```python
from build123d import *

# Parameters (mm, degrees)
SKETCH1_R           = 50
BOSS_EXTRUDE2_DEPTH = 10
SKETCH7_R           = 10.430903113
CUT_EXTRUDE5_DEPTH  = 10
CUT_EXTRUDE8_DEPTH  = 72.414284285
CUT_EXTRUDE9_DEPTH  = 72.414284285
CIRPATTERN3_COUNT   = 9
CIRPATTERN3_ANGLE   = 88
CIRPATTERN4_COUNT   = 17
CIRPATTERN4_ANGLE   = 176
SCALE3_SCALE        = 0.75
BOSS_EXTRUDE3_DEPTH = 15
BOSS_EXTRUDE6_DEPTH = 25
SKETCH19_R          = 1.5
CUT_EXTRUDE10_DEPTH = 2.5


with BuildPart() as part:
    # Sketch1 → Boss-Extrude2 (new body)
    with BuildSketch(Plane.YZ):
        with Locations(Location((0, 0, 0), (0, 0, 270))):
            Circle(SKETCH1_R)
    extrude(amount=BOSS_EXTRUDE2_DEPTH)

    # Sketch7 → Cut-Extrude5 (cut)
    with BuildSketch(Plane.YZ.offset(10)):
        with Locations(Location((0, 0, 0), (0, 0, 270))):
            Circle(SKETCH7_R)
    extrude(amount=-CUT_EXTRUDE5_DEPTH, mode=Mode.SUBTRACT)

    # Sketch10 → Cut-Extrude8 (cut, through all)
    with BuildSketch(Plane.YZ.offset(10)):
        with BuildLine():
            Line((-43.954399928, 0), (-14.132830655, 0))
            ThreePointArc((-14.132830655, 0), (10.058249892, -10.149932648), (0.129658997, 14.132830655))
            Line((0.129658997, 14.132830655), (0, 44.213717922))
            ThreePointArc((0, 44.213717922), (31.393478761, -30.950795255), (-43.954399928, 0))
        make_face()
    extrude(amount=-CUT_EXTRUDE8_DEPTH, mode=Mode.SUBTRACT)

    # Sketch12 → Cut-Extrude9 (cut, through all)
    with BuildSketch(Plane.YZ.offset(10)):
        Polygon((47.400317311, 0), (47.400317311, 0.608013975), (44.136400392, 2.742660057), (44.128376975, -2.615132262), (47.400317311, -0.500577082), align=None)
    cut_extrude9 = extrude(amount=-CUT_EXTRUDE9_DEPTH, mode=Mode.SUBTRACT)

    # CirPattern3: Cut-Extrude9 ×9 about axis
    cirpattern3_axis = Axis((0, 0.129658997, 0.129658997), (1, 0, 0))
    for i in range(1, CIRPATTERN3_COUNT):
        add(cut_extrude9.rotate(cirpattern3_axis, i * CIRPATTERN3_ANGLE / (CIRPATTERN3_COUNT - 1)), mode=Mode.SUBTRACT)

    # CirPattern4: Cut-Extrude9 ×17 about axis
    cirpattern4_axis = Axis((0, 0.129658997, 0.129658997), (-1, 0, 0))
    for i in range(1, CIRPATTERN4_COUNT):
        add(cut_extrude9.rotate(cirpattern4_axis, i * CIRPATTERN4_ANGLE / (CIRPATTERN4_COUNT - 1)), mode=Mode.SUBTRACT)


with BuildPart() as part_1:
    # Scale3: scaled about (0, 0, 0)
    add(part.part.scale(SCALE3_SCALE))

    # Sketch15 → Boss-Extrude3 (add)
    with BuildSketch(Plane.YZ.offset(7.5)):
        Polygon((-12.172757091, 41.059305133), (-7.956454872, 36.843002914), (-36.24072612, 8.558731667), (-40.457028339, 12.775033886), align=None)
    extrude(amount=BOSS_EXTRUDE3_DEPTH)

    # Sketch20 → Boss-Extrude6 (add)
    with BuildSketch(Plane(origin=(7.5, 0, 0), x_dir=(0, -1, 0), z_dir=(-1, 0, 0))):
        Polygon((7.956454872, 36.843002914), (12.172757091, 41.059305133), (40.457028339, 12.775033886), (36.24072612, 8.558731667), align=None)
    extrude(amount=BOSS_EXTRUDE6_DEPTH)

    # Sketch19 → Cut-Extrude10 (cut)
    with BuildSketch(Plane(origin=(0, -26.616031112, 26.616031112), x_dir=(1, 0, 0), z_dir=(0, -0.7071067811865476, 0.7071067811865475))):
        with Locations(Location((-14.5, -16.574125994, 0), (0, 0, 270))):
            Circle(SKETCH19_R)
        with Locations(Location((-14.5, 17.425874006, 0), (0, 0, 270))):
            Circle(SKETCH19_R)
        with Locations(Location((-11.5, 14.425874006, 0), (0, 0, 270))):
            Circle(SKETCH19_R)
        with Locations(Location((-11.5, -13.574125994, 0), (0, 0, 270))):
            Circle(SKETCH19_R)
        with Locations(Location((19.5, 17.425874006, 0), (0, 0, 270))):
            Circle(SKETCH19_R)
        with Locations(Location((16.5, 14.425874006, 0), (0, 0, 270))):
            Circle(SKETCH19_R)
        with Locations(Location((16.5, -13.574125994, 0), (0, 0, 270))):
            Circle(SKETCH19_R)
        with Locations(Location((19.5, -16.574125994, 0), (0, 0, 270))):
            Circle(SKETCH19_R)
    extrude(amount=-CUT_EXTRUDE10_DEPTH, mode=Mode.SUBTRACT)


solid = part_1.part
```
Design review of the part built by this model. Coordinates are the model's own, in mm. A direction names the side the tool comes from. Coordinates: 2 decimals unless noted, no trailing zeros. Order: outer loops, then holes, each group sorted by start corner. A loop starts at its lowest first (then second) coordinate and runs counter-clockwise, first axis right, second up. Notation, with made-up numbers: (4.5, -21) -> (61.5, -21) arc R4 ccw to (61.5, -17) -> close; hole circle Ø8 at (56, 21.25). An arc over 180 degrees is marked (long way). One line per item, written item: value. Start each with the question number.
Q1. Mouldability with a two-part tool opening along X and no side actions: class faces 3 (the cylindrical face through (16.951, -16.556, 34.933)), 4 (the flat face through (3.802, 33.434, -7.683)) as pulls with the +X half, pulls with the -X half, needs draft (parallel to the pull), parting line crosses it, or undercut.
Q2. For probe 1 along Y at (x, z) = (2, -5.5); probe 2 along X at (y, z) = (31, -19.5); probe 3 along Y at (x, z) = (8.5, 13.5), list the stretches that pass through material, from the lowest coordinate up.
Q3. Take a section at B-B, the plane x = 2. Give the number of separate pieces and of enclosed holes in the cut face, then the cut area to 3 significant figures.
Q4. Insertion check: pin 1 Ø3 at (y, z) = (20, -25.5) entering from -X; pin 2 Ø6 at (x, y) = (-3.5, -16) entering from -Z; pin 3 Ø3 at (x, y) = (2.5, -25) entering from +Z. Each pin has a flat end and moves straight along its axis. Give the tip position at first contact, or say it passes through.
Q5. Take a section at A-A, the plane x = -7.5. State the section outline as (y, z) points, then the cut area to 3 significant figures.
Q6. Tool access review of faces 1 (the flat face through (3.802, 15.075, -30.721)), 2 (the flat face through (-14.479, -12.511, 37.185)): name each direction out of +Z, -Z, +X, -X, +Y, -Y from which nothing blocks a thin tool from reaching the whole face with its end or side.
Values follow:
1. face 3: undercut
1. face 4: needs draft
2. probe 1: y = -37.09 to -32.49, -9.1 to -5.56, 5.56 to 9.2, 34.13 to 37.09
2. probe 2: x = 0 to 7.5
2. probe 3: y = -39.73 to -31.3
3. separate pieces: 1
3. enclosed holes: 2
3. area: 1,850 mm2
4. pin 1: stops at x = 0
4. pin 2: stops at z = 25.8
4. pin 3: stops at z = 29.73
5. outline: (-40.46, 12.78) -> (-36.24, 8.56) -> (-7.96, 36.84) -> (-12.17, 41.06) -> close
5. area: 239 mm2
6. face 1: +X, -X
6. face 2: none
